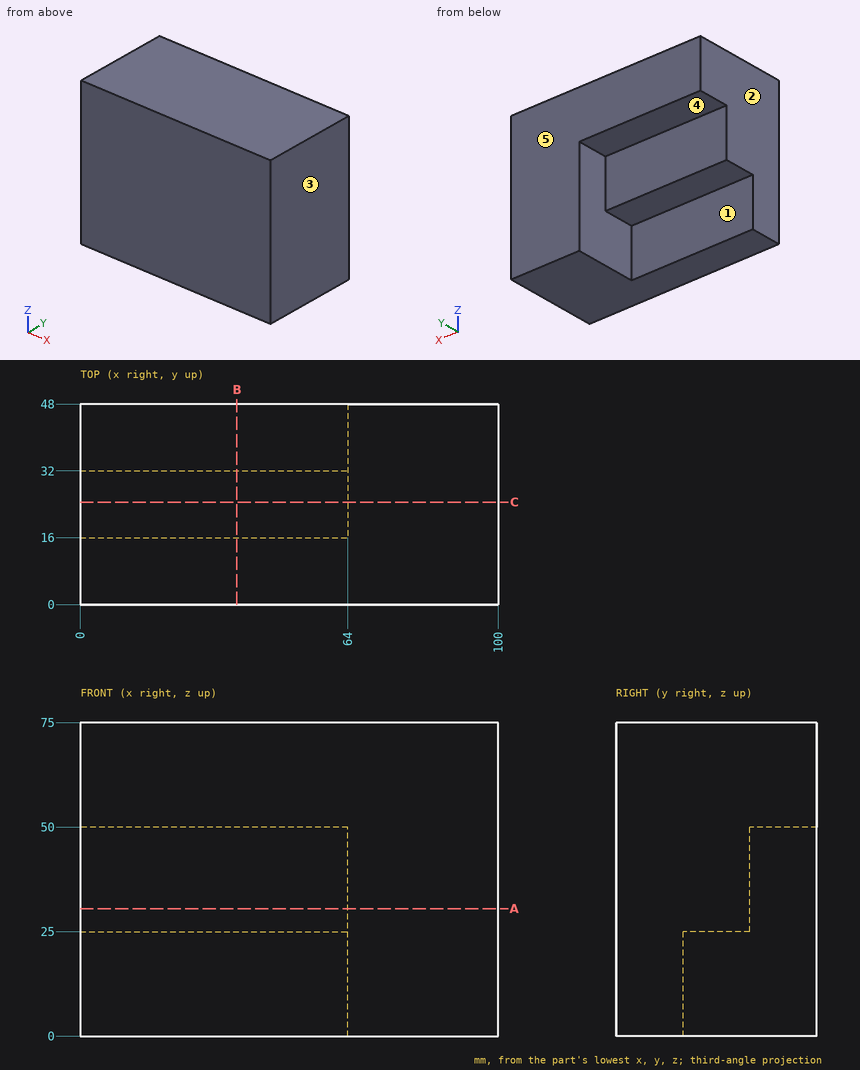
Print and shaded views of the part. All mm, measured from the part's lowest x, y and z. A direction names the side the tool comes from. Coordinates: 2 decimals unless noted, no trailing zeros. Loops run counter-clockwise (first coordinate to the right, second up) from the corner with the lowest first, then second, coordinate; pieces in that order, holes last. Notation, with made-up numbers: (-6.75, 88) -> (44.25, 88) arc R16 ccw to (44.25, 105) -> close; hole circle Ø8 at (-26, 46.25). An arc over 180 degrees is marked (long way). Use a Markdown table: item, result. Add a question column.
Item 1: Probe probe 1 along Y at (x, z) = (63, 45); probe 2 along Y at (x, z) = (52, 24); probe 3 along Z at (x, y) = (14, 45.5). List the from-to ranges inside material, lowest first.
Item 2: Band-saw the part on A-A on z = 30.5. Write the cut outline in (x, y).
Item 3: Which spindle directions (+Z, -Z, +X, -X, +Y, -Y) get a long thin tool onto all of the face, cutting with end or side? Do the marked faces 4 and 5. Say none if no direction does.
Item 4: Pull direction X, two halves, no side cores. Call the marked faces 1, 2 and 3: +X half, -X half, draft (parallel to the pull), parting line (faces both ways), or undercut.
Item 5: Flat gauge pins, fed straight in: P1, Ø8, axis at x = 33.5, y = 41.5, coming from the -Z side; P2, Ø1.5, axis at x = 60, z = 12.5, coming from the +Y side; P3, Ø5, axis at x = 20.5, y = 26, coming from the -Z side; P4, Ø4, axis at x = 89.5, y = 40.5, coming from the -Z side. Where does each tip first touch, or does it go through?
Item 6: Band-saw the part on C-C on y = 24.5. Write the cut outline in (x, z), plus the area to 3 significant figures.
Item 7: Band-saw the part on B-B on x = 37.5. Write the cut outline in (y, z).
Geometry says:
| question | item | result |
|---|---|---|
| 1 | probe 1 | 0 to 32 |
| 1 | probe 2 | 0 to 16 |
| 1 | probe 3 | 50 to 75 |
| 2 | outline | (0, 0) -> (100, 0) -> (100, 48) -> (64, 48) -> (64, 32) -> (0, 32) -> close |
| 3 | face 4 | -Z, -X, +Y |
| 3 | face 5 | +Z, -Z, +X, -X, +Y |
| 4 | face 1 | draft |
| 4 | face 2 | -X half |
| 4 | face 3 | +X half |
| 5 | P1 | z = 50 |
| 5 | P2 | y = 16 |
| 5 | P3 | z = 25 |
| 5 | P4 | z = 0 |
| 6 | outline | (0, 25) -> (64, 25) -> (64, 0) -> (100, 0) -> (100, 75) -> (0, 75) -> close |
| 6 | area | 5,900 mm² |
| 7 | outline | (0, 0) -> (16, 0) -> (16, 25) -> (32, 25) -> (32, 50) -> (48, 50) -> (48, 75) -> (0, 75) -> close |
